Here's how the part is built. I have some questions about the finished solid (model axes, mm). Round coordinates to 2 decimals unless told otherwise and drop trailing zeros. Write each loop counter-clockwise with the first axis right and the second up, starting at its lowest first coordinate (ties: lowest second). Pieces come first, ordered by that corner, then holes. Notation, with made-up numbers: (45, -22) - (94, -22) arc R11 ccw to (94, -1) - close; hole circle Ø5 at (61.25, -17.75). An arc over 180 degrees is marked (long way). Write item = value, one per line. Start each with the question number.
Item 1: If we section it at C-C (y = 3): Please give me the cut outline in (x, z).
Item 2: If we section it at B-B (x = 34): Please give me the cut outline in (y, z), and give its area (3 significant figures).
Item 3: If I drill on line 1 along Z through (x, y) = (27, 5.5); line 2 along Y through (x, z) = (10, 1); line 3 along X through (y, z) = (0.75, -19.5), over which ranges is the centre line in solid material (lowest first)? Write a range as [from, to].
Item 4: For P1, Ø2.5, axis at x = 5.5, z = 1.5, coming from the +Y side, with a flat end and sliding along its axis, tell me the tip position at first contact or that it passes through.
Item 5: If we section it at A-A (y = 7.75): Please give me the cut outline in (x, z).
Item 6: If we section it at D-D (z = 16): Please give me the cut outline in (x, y).
```python
from build123d import *

# Parameters (mm, degrees)
SKETCH1_W           = 100
SKETCH1_H           = 50
BOSS_EXTRUDE1_DEPTH = 10
CHAMFER1_SIZE       = 10
SKETCH2_W           = 113.165724781
SKETCH2_H           = 8
CUT_EXTRUDE1_DEPTH  = 5


with BuildPart() as part:
    # Sketch1 → Boss-Extrude1 (new body)
    with BuildSketch(Plane(origin=(0, 0, 0), x_dir=(1, 0, 0), z_dir=(0, 1, 0))):
        Rectangle(SKETCH1_W, SKETCH1_H)
    extrude(amount=BOSS_EXTRUDE1_DEPTH)

    # Chamfer1
    chamfer1_edges = [part.edges().sort_by_distance(p)[0] for p in [
        (-50, 5, -25),
        (50, 5, -25),
        (50, 5, 25),
        (-50, 5, 25),
    ]]
    chamfer(chamfer1_edges, length=CHAMFER1_SIZE)

    # Sketch2 → Cut-Extrude1 (cut)
    with BuildSketch(Plane(origin=(0, 10, 0), x_dir=(1, 0, 0), z_dir=(0, 1, 0))):
        with Locations((-1.797960114, 0)):
            Rectangle(SKETCH2_W, SKETCH2_H)
    extrude(amount=-CUT_EXTRUDE1_DEPTH, mode=Mode.SUBTRACT)


solid = part.part
```
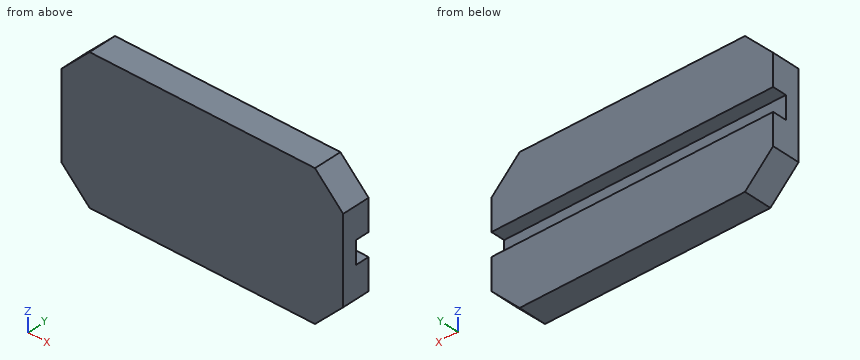
Reply:
q1.outline = (-50, -15) - (-40, -25) - (40, -25) - (50, -15) - (50, 15) - (40, 25) - (-40, 25) - (-50, 15) - close
q2.outline = (0, -25) - (10, -25) - (10, -4) - (5, -4) - (5, 4) - (10, 4) - (10, 25) - (0, 25) - close
q2.area = 460 mm2
q3.line_1 = [-25, -4], [4, 25]
q3.line_2 = [0, 5]
q3.line_3 = [-45.5, 45.5]
q4.P1 = 5
q5.outline = (-50, -15) - (-40, -25) - (40, -25) - (50, -15) - (50, -4) - (-50, -4) - close; (-50, 4) - (50, 4) - (50, 15) - (40, 25) - (-40, 25) - (-50, 15) - close
q6.outline = (-49, 0) - (49, 0) - (49, 10) - (-49, 10) - close
